Autodesk Fusion 360 part; units mm, degrees
sketch "Hex Polygon" plane through (0, 0, 0) normal (0, 0, 1) x (1, 0, 0)
  line L0 (5.7735, 10) -> (-5.7735, 10)
  line L1 (-5.7735, 10) -> (-11.547, 0)
  line L2 (-11.547, 0) -> (-5.7735, -10)
  line L3 (-5.7735, -10) -> (5.7735, -10)
  line L4 (5.7735, -10) -> (11.547, 0)
  line L5 (11.547, 0) -> (5.7735, 10)
  dimension "d1" = 10
extrude "Extrude1" add sketch "Hex Polygon" along normal blind 10
sketch "Chamfer Sketch" plane through (0, 0, 0) normal (0, 1, 0) x (1, 0, 0)
  line L0 (11.547, -10) -> (10.047, -10)
  line L1 (10.047, -10) -> (11.547, -8.5)
  line L2 (11.547, -8.5) -> (11.547, -10)
  point P0 (11.547, -10)
  dimension "d4" = 1.5
revolve "Revolve1" cut sketch "Chamfer Sketch" angle 360 about axis through (0, 0, 1.75) along (0, 0, 1)
hole "Hole1" at (0, 0, 10) direction (0, 0, -1) diameter 11.035 end through all countersink diameter 14 countersink angle 90
ref_plane "WorkPlane1" through (0, 0, 5) normal (0, 0, 1) x (1, 0, 0)
mirror "Mirror1" about plane through (0, 0, 5) normal (0, 0, 1) of "Revolve1", "Hole1"
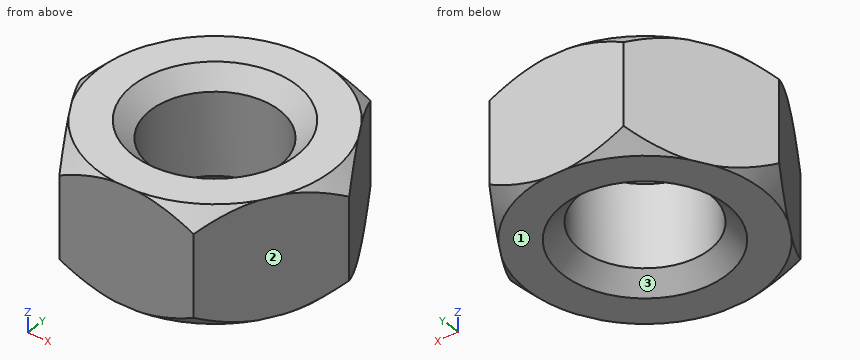
The model under review builds one solid part; all positions refer to its coordinate system, in mm. Face numbers are marked on the shaded views. Give positions to 0.01 mm unless a question says otherwise; leave off trailing zeros. Loops run counter-clockwise (first coordinate to the right, second up) from the corner with the lowest first, then second, coordinate; pieces in that order, holes last. Notation, with made-up numbers: (-32, 59.25) -> (-3, 59.25) arc R21 ccw to (-3, 88.25) -> close; hole circle Ø10 at (19.5, 30). An arc over 180 degrees is marked (long way). Put each result on its own line as item: value. Start each with the question number.
1. We need section D-D on x = 8.75. State the section outline as (y, z) points.
2. We need section C-C on z = 9.5. State the section outline as (x, y) points, then the cut area to 3 significant figures.
3. Wall thickness on probe 1 along Y at (x, z) = (0, 6); probe 2 along X at (y, z) = (-3.5, 7.25); probe 3 along X at (y, z) = (1.5, 0.75): over which ranges is each line inside the solid? List them lowest first.
4. We need section A-A on x = 0. State the section outline as (y, z) points, then the cut area to 3 significant figures.
5. We need section B-B on z = 4.5. State the section outline as (x, y) points (1 decimal).
6. Mouldability with a two-part tool opening along Y and no side actions: class the marked faces 1, 2 and 3 as released by +Y, released by -Y, zero draft, split by the parting line, or undercut.
7. Clearance check with flat-ended pins moving along their axes: P1, Ø1, axis at y = -3, z = 5.5, coming from the +X side; P2, Ø1, axis at y = -4, z = 7.5, coming from the -X side. State where each tip first meets the part, or that it passes through.
Determined:
1. outline: (-4.84, 0) -> (4.84, 0) -> (4.84, 10) -> (-4.84, 10) -> close
2. outline: (-10.34, -2.1) -> (-6.98, -7.9) arc R10.55 ccw to (-3.35, -10) -> (3.35, -10) arc R10.55 ccw to (6.98, -7.9) -> (10.34, -2.1) arc R10.55 ccw to (10.34, 2.1) -> (6.98, 7.9) arc R10.55 ccw to (3.35, 10) -> (-3.35, 10) arc R10.55 ccw to (-6.98, 7.9) -> (-10.34, 2.1) arc R10.55 ccw to start; hole circle Ø13 at (0, 0)
2. area: 202 mm^2
3. probe 1: -10 to -5.52, 5.52 to 10
3. probe 2: -9.53 to -4.27, 4.27 to 9.53
3. probe 3: -10.68 to -6.07, 6.07 to 10.68
4. outline: (-10, 0) -> (-7, 0) -> (-5.52, 1.48) -> (-5.52, 8.52) -> (-7, 10) -> (-10, 10) -> close; (5.52, 1.48) -> (7, 0) -> (10, 0) -> (10, 10) -> (7, 10) -> (5.52, 8.52) -> close
4. area: 85.3 mm^2
5. outline: (-11.5, 0) -> (-5.8, -10) -> (5.8, -10) -> (11.5, 0) -> (5.8, 10) -> (-5.8, 10) -> close; hole circle Ø11 at (0, 0)
6. face 1: zero draft
6. face 2: released by -Y
6. face 3: undercut
7. P1: x = 10.1
7. P2: x = -9.53
